```python
from build123d import *

# Parameters (mm, degrees)
SKETCH2_W                  = 132
SKETCH2_H                  = 232
PLATE_SIZE_DEPTH           = 4.4
SKETCH4_OUTSIDE_W          = 187.392
SKETCH4_OUTSIDE_H          = 287.392
OUTER_PROFILE_DEPTH        = 5.4
M3_CLEARANCE_HOLE1_D       = 3.5
F_18_0_18_DIAMETER_HOLE4_D = 18
M3_CLEARANCE_HOLE2_D       = 3.5
M3_CLEARANCE_HOLE3_D       = 3
M3_CLEARANCE_HOLE4_D       = 3
SKETCH17_R                 = 9.017
CUT_EXTRUDE1_DEPTH         = 53.34


with BuildPart() as part:
    # Sketch2 → Plate Size (new body)
    with BuildSketch(Plane(origin=(0, 0, 0), x_dir=(1, 0, 0), z_dir=(0, 1, 0))):
        Rectangle(SKETCH2_W, SKETCH2_H)
    extrude(amount=PLATE_SIZE_DEPTH)

    # Sketch4 outside → Outer Profile (cut, through all)
    with BuildSketch(Plane(origin=(0, 0, 0), x_dir=(1, 0, 0), z_dir=(0, 1, 0))):
        Rectangle(SKETCH4_OUTSIDE_W, SKETCH4_OUTSIDE_H)
        with BuildLine():
            Line((-64.599996007, 76), (-47, 76))
            Line((-47, 76), (-47, 4))
            Line((-47, 4), (-62, 4))
            ThreePointArc((-62, 4), (-66, 0), (-62, -4))
            Line((-62, -4), (-47, -4))
            Line((-47, -4), (-47, -76))
            Line((-47, -76), (-64.599996007, -76))
            ThreePointArc((-64.599996007, -76), (-65.462483305, -76.493921289), (-65.472968926, -77.487768677))
            ThreePointArc((-65.472968926, -77.487768677), (0, -115.905117871), (65.472968926, -77.487768677))
            ThreePointArc((65.472968926, -77.487768677), (65.462483305, -76.493921289), (64.599996007, -76))
            Line((64.599996007, -76), (47, -76))
            Line((47, -76), (47, -4))
            Line((47, -4), (62, -4))
            ThreePointArc((62, -4), (66, 0), (62, 4))
            Line((62, 4), (47, 4))
            Line((47, 4), (47, 76))
            Line((47, 76), (64.599996007, 76))
            ThreePointArc((64.599996007, 76), (65.462483305, 76.493921289), (65.472968926, 77.487768677))
            ThreePointArc((65.472968926, 77.487768677), (0, 115.905117871), (-65.472968926, 77.487768677))
            ThreePointArc((-65.472968926, 77.487768677), (-65.462483305, 76.493921289), (-64.599996007, 76))
        make_face(mode=Mode.SUBTRACT)
    extrude(amount=OUTER_PROFILE_DEPTH, mode=Mode.SUBTRACT)

    # M3 Clearance Hole1 (through all)
    with Locations(Plane.XZ):
        with Locations((-55.999996141, 80.000001937), (55.999996141, 80.000001937), (-52.5, -85), (52.5, -85), (-55.999996141, 0), (55.999996141, 0)):
            Hole(M3_CLEARANCE_HOLE1_D / 2)

    # Ø18.0 (18) Diameter Hole4 (through all)
    with Locations(Plane.XZ):
        with Locations((0, -56), (0, 56)):
            Hole(F_18_0_18_DIAMETER_HOLE4_D / 2)

    # M3 Clearance Hole2 (through all)
    with Locations(Plane.XZ):
        with Locations((18.75, -18.75), (-18.75, 18.75), (18.75, 18.75), (-18.75, -18.75)):
            Hole(M3_CLEARANCE_HOLE2_D / 2)

    # M3 Clearance Hole3 (through all)
    with Locations(Plane.XZ):
        with Locations((-25.5, -66.00000008), (25.5, 65.00000008), (-25.5, 65.00000008), (25.5, -66.00000008), (-25.5, -58.00000008), (25.5, -58.00000008), (25.5, 57.00000008), (-25.5, 57.00000008)):
            Hole(M3_CLEARANCE_HOLE3_D / 2)

    # M3 Clearance Hole4 (through all)
    with Locations(Plane.XZ):
        with Locations((-20, -107), (20, -107), (-20, -82), (20, -82)):
            Hole(M3_CLEARANCE_HOLE4_D / 2)

    # Sketch17 → Cut-Extrude1 (cut)
    with BuildSketch(Plane(origin=(0, 4.4, 0), x_dir=(1, 0, 0), z_dir=(0, 1, 0))):
        Circle(SKETCH17_R)
    extrude(amount=-CUT_EXTRUDE1_DEPTH, mode=Mode.SUBTRACT)


solid = part.part
```
Part model, mm, in its own coordinate system. A direction names the side the tool comes from. Coordinates: 2 decimals unless noted, no trailing zeros. Write each loop counter-clockwise with the first axis right and the second up, starting at its lowest first coordinate (ties: lowest second). Pieces come first, ordered by that corner, then holes.
Item 1: Which spindle directions (+Z, -Z, +X, -X, +Y, -Y) get a long thin tool onto all of the face, cutting with end or side? Do faces 1 (the face through (56, 2, 76)), 2 (the face through (-47, 2, -41)), 3 (the face through (1.114, 2.169, -115.897)). Say none if no direction does.
Item 2: Slice it at D-D (x = -35). Write the cut outline in (y, z), and give its area (3 significant figures).
Item 3: Slice it at C-C (z = 12). Write the cut outline in (x, y).
Item 4: Slice it at B-B (y = 1.05). Count the separate pieces of the cut face and the enclosed holes in it, and give its area (3 significant figures).
Item 5: Slice it at A-A (x = 0.5). Write the cut outline in (y, z), and give its area (3 significant figures).
Item 6: Mould opens along X. For faces 4 (the face through (56, 2, -76)), 5 (the face through (-47, 2, 39)), 6 (the face through (-1.955, 2.231, 8.803)) say: released by +X, released by -X, zero draft, split by the parting line, or undercut.
Item 7: Probe line 1 (Z direction, x = 0, y = 2.4); line 2 (Z direction, x = 52.5, y = 2.5); line 3 (Z direction, x = -20, y = 3.35). List the from-to ranges inside material, lowest first.
Item 8: Pin check, flat tips, straight feed: pin 1 (6 mm diameter, centred on x = 46, z = 9.5, fed in from -Y); pin 2 (2 mm diameter, centred on x = 54, y = 3, fed in from -Z); pin 3 (1 mm diameter, centred on y = 0.5, z = 47.5, fed in from -X); pin 4 (1.3 mm diameter, centred on x = 57.5, y = 1.5, fed in from +Z). Stop position of each tip, or through.
Results found:
1. face 1: +X, +Y, -Y
1. face 2: -X, +Y, -Y
1. face 3: -Z, +Y, -Y
2. outline: (0, -107.24) - (4.4, -107.24) - (4.4, 107.24) - (0, 107.24) - close
2. area: 944 mm2
3. outline: (-47, 0) - (47, 0) - (47, 4.4) - (-47, 4.4) - close
4. separate pieces: 1
4. enclosed holes: 25
4. area: 21,200 mm2
5. outline: (0, -115.9) - (4.4, -115.9) - (4.4, -64.99) - (0, -64.99) - close; (0, -47.01) - (4.4, -47.01) - (4.4, -9) - (0, -9) - close; (0, 9) - (4.4, 9) - (4.4, 47.01) - (0, 47.01) - close; (0, 64.99) - (4.4, 64.99) - (4.4, 115.9) - (0, 115.9) - close
5. area: 783 mm2
6. face 4: zero draft
6. face 5: released by -X
6. face 6: undercut
7. line 1: z = -115.91 to -65, -47 to -9.02, 9.02 to 47, 65 to 115.91
7. line 2: z = -94.47 to -86.75, -83.25 to -76, -4 to 4, 76 to 94.47
7. line 3: z = -113.19 to -108.5, -105.5 to -83.5, -80.5 to -19.97, -17.53 to 17.53, 19.97 to 113.19
8. pin 1: stops at y = 0
8. pin 2: stops at z = -93.97
8. pin 3: stops at x = -47
8. pin 4: stops at z = 89.82
